The model under review builds one solid part; all positions refer to its coordinate system, in mm. A direction names the side the tool comes from. Round coordinates to 2 decimals unless told otherwise and drop trailing zeros. Write each loop counter-clockwise with the first axis right and the second up, starting at its lowest first coordinate (ties: lowest second). Pieces come first, ordered by that corner, then holes. Notation, with made-up numbers: (47, 10) -> (86, 10) arc R20 cw to (86, 16) -> close; hole circle Ø5 at (-15.5, 68.5). An arc over 180 degrees is marked (long way). Answer as a JSON object with one key per item and string values. Group by question number.
1) Machinability: for faces 4 (the cylindrical face through (30, 0, 5)), 5 (the flat face through (-55, 15, 45)), 6 (the flat face through (-55, -22, 60)), 7 (the flat face through (-1, 14, 10)), which of the approach directions +Z, -Z, +X, -X, +Y, -Y give a long, thin tool a straight path to every point of the face, cutting with its end or side? Answer none if there is none.
2) To check wall thickness, follow probe 1 along Z at (x, y) = (78, -21); probe 2 along X at (y, z) = (-25.5, 36.5); probe 3 along Z at (x, y) = (47, -11). State the ranges of each line that lie inside material, in increasing order. Write a range as [from, to].
3) Mouldability with a two-part tool opening along X and no side actions: class faces 1 (the cylindrical face through (123.17, 0.66, 78.24)), 2 (the flat face through (77, 0, 37)), 3 (the cylindrical face through (-55, 0, 15)) as pulls with the +X half, pulls with the -X half, needs draft (parallel to the pull), parting line crosses it, or undercut.
4) We need section D-D, the plane y = 20. Write out the cut boundary in (x, z).
5) We need section A-A, the plane z = 33.5. Write out the cut boundary in (x, y), then the cut area to 3 significant figures.
6) We need section C-C, the plane x = -12. Write out the cut boundary in (y, z).
7) Insertion check: pin 1 Ø4 at (x, y) = (-27, -7) entering from +Z; pin 2 Ø8 at (x, y) = (-55.5, 25) entering from +Z; pin 3 Ø4 at (x, z) = (96, 69) entering from +Y. Each pin has a flat end and moves straight along its axis. Give the tip position at first contact, or say it passes through.
8) We need section B-B, the plane y = -3. Write out the cut boundary in (x, z), then the cut area to 3 significant figures.
from build123d import *

# Parameters (mm, degrees)
SKETCH1_W           = 100
SKETCH1_H           = 60
BOSS_EXTRUDE1_DEPTH = 10
BOSS_EXTRUDE2_DEPTH = 10
BOSS_EXTRUDE3_DEPTH = 60
SKETCH5_R           = 25
SKETCH5_R_2         = 15
BOSS_EXTRUDE4_DEPTH = 20
CUT_EXTRUDE3_DEPTH  = 20
CUT_EXTRUDE4_START  = -20
SKETCH6_R           = 15
CUT_EXTRUDE4_DEPTH  = 20


with BuildPart() as part:
    # Sketch1 → Boss-Extrude1 (new body)
    with BuildSketch(Plane.XY):
        Rectangle(SKETCH1_W, SKETCH1_H)
        with BuildLine():
            Line((-10, 10), (20, 10))
            ThreePointArc((20, 10), (30, 0), (20, -10))
            Line((20, -10), (-10, -10))
            ThreePointArc((-10, -10), (-20, 0), (-10, 10))
        make_face(mode=Mode.SUBTRACT)
    extrude(amount=BOSS_EXTRUDE1_DEPTH)

    # Sketch3 → Boss-Extrude2 (add)
    with BuildSketch(Plane.ZY.offset(50)):
        with BuildLine():
            Line((0, 30), (60, 30))
            Line((60, 30), (60, 15))
            Line((60, 15), (30, 15))
            ThreePointArc((30, 15), (15, 0), (30, -15))
            Line((30, -15), (60, -15))
            Line((60, -15), (60, -30))
            Line((60, -30), (0, -30))
            Line((0, -30), (0, 30))
        make_face()
    extrude(amount=BOSS_EXTRUDE2_DEPTH)

    # Sketch4 → Boss-Extrude3 (add)
    with BuildSketch(Plane.XZ.offset(30)):
        Polygon((50, 10), (125, 85), (130, 80), (50, 0), align=None)
    extrude(amount=-BOSS_EXTRUDE3_DEPTH)

    # Sketch5 → Boss-Extrude4 (add)
    with BuildSketch(Plane(origin=(20, 0, -20), x_dir=(0.7071067811865462, 0, 0.7071067811865488), z_dir=(-0.7071067811865488, 0, 0.7071067811865462))):
        with Locations((112.426406871, 0)):
            Circle(SKETCH5_R)
        with Locations((112.426406871, 0)):
            Circle(SKETCH5_R_2, mode=Mode.SUBTRACT)
    extrude(amount=BOSS_EXTRUDE4_DEPTH)

    # Sketch5<4> → Cut-Extrude3 (cut)
    with BuildSketch(Plane(origin=(20, 0, -20), x_dir=(0.7071067811865462, 0, 0.7071067811865488), z_dir=(-0.7071067811865488, 0, 0.7071067811865462))):
        with BuildLine():
            Line((112.426406871, -30), (148.492424049, -30))
            Line((148.492424049, -30), (148.492424049, 30))
            Line((148.492424049, 30), (112.426406871, 30))
            ThreePointArc((112.426406871, 30), (142.426406871, 0), (112.426406871, -30))
        make_face()
    extrude(amount=-CUT_EXTRUDE3_DEPTH, mode=Mode.SUBTRACT)

    # Sketch6 → Cut-Extrude4 (cut)
    with BuildSketch(Plane(origin=(20, 0, -20), x_dir=(0.7071067811865464, 0, 0.7071067811865488), z_dir=(-0.7071067811865488, 0, 0.7071067811865464)).offset(CUT_EXTRUDE4_START)):
        with Locations(Location((112.426406871, 0, 0), (0, 0, 180))):
            Circle(SKETCH6_R)
    extrude(amount=CUT_EXTRUDE4_DEPTH, mode=Mode.SUBTRACT)


solid = part.part
Here are the results:
{
 "1": {"face 4": "+Z, -Z", "face 5": "+Z, -X", "face 6": "+Z, -X, +Y, -Y", "face 7": "+Z, +Y, -Y"},
 "2": {"probe 1": "z = [28, 38], [61.81, 66.28]", "probe 2": "x = [-60, -50], [76.5, 86.5]", "probe 3": "z = [0, 10]"},
 "3": {"face 1": "pulls with the +X half", "face 2": "undercut", "face 3": "needs draft"},
 "4": {"outline": "(-60, 0) -> (50, 0) -> (120.31, 70.31) -> (115.31, 75.31) -> (110.1, 70.1) -> (95.96, 84.25) -> (74.75, 63.03) -> (88.89, 48.89) -> (50, 10) -> (-50, 10) -> (-50, 60) -> (-60, 60) -> close"},
 "5": {"outline": "(-60, -30) -> (-50, -30) -> (-50, -15) -> (-60, -15) -> close; (-60, 15) -> (-50, 15) -> (-50, 30) -> (-60, 30) -> close; (73.5, -30) -> (83.5, -30) -> (83.5, 30) -> (73.5, 30) -> close", "area": "900 mm^2"},
 "6": {"outline": "(-30, 0) -> (-9.8, 0) -> (-9.8, 10) -> (-30, 10) -> close; (9.8, 0) -> (30, 0) -> (30, 10) -> (9.8, 10) -> close"},
 "7": {"pin 1": "stops at z = 10", "pin 2": "stops at z = 60", "pin 3": "stops at y = 24.9"},
 "8": {"outline": "(-60, 0) -> (-19.54, 0) -> (-19.54, 10) -> (-50, 10) -> (-50, 15.3) -> (-60, 15.3) -> close; (29.54, 0) -> (50, 0) -> (94.11, 44.11) -> (74.96, 63.25) -> (67.81, 56.09) -> (81.95, 41.95) -> (50, 10) -> (29.54, 10) -> close; (95.75, 84.03) -> (114.89, 64.89) -> (125.6, 75.6) -> (120.6, 80.6) -> (117.05, 77.05) -> (102.91, 91.19) -> close", "area": "1,590 mm^2"}
}
